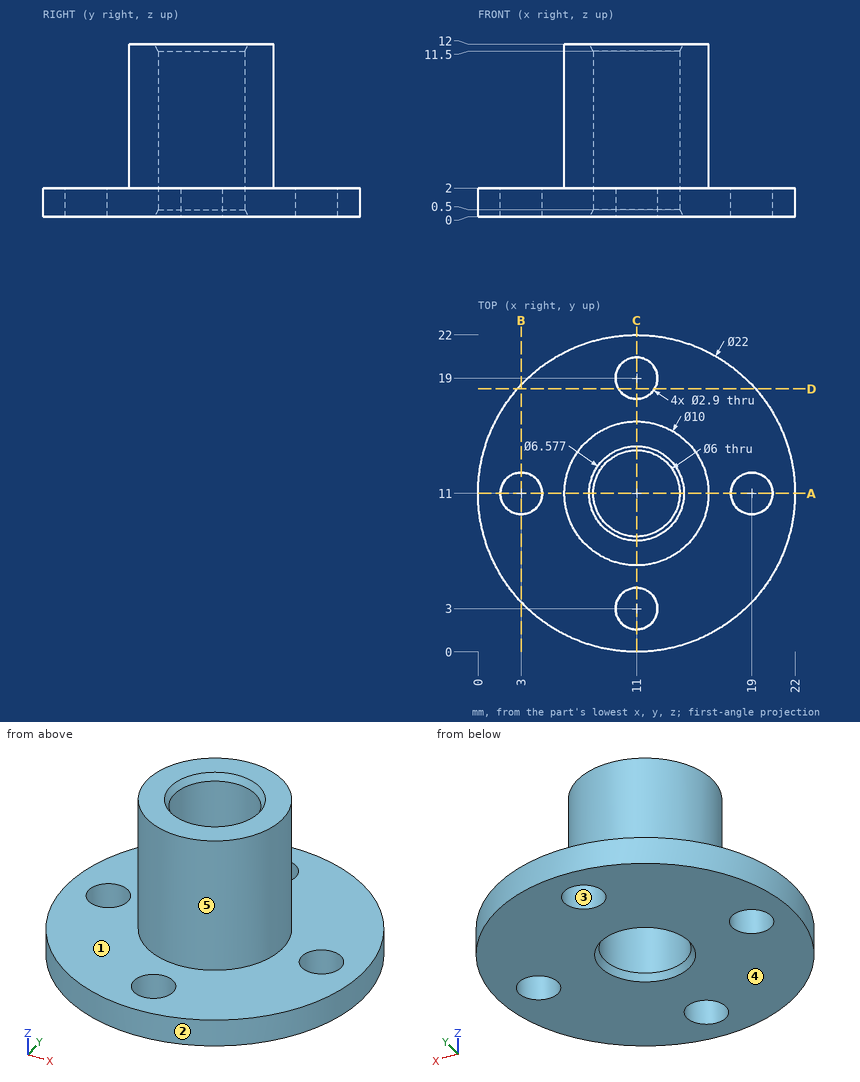
Can you work these out from the drawing? Everything is in mm from the part's minimum corner. A direction names the side the tool comes from. Coordinates: 2 decimals unless noted, no trailing zeros. Write each loop counter-clockwise with the first axis right and the second up, starting at its lowest first coordinate (ties: lowest second). Pieces come first, ordered by that corner, then holes. Notation, with made-up numbers: (23, 75.5) -> (54, 75.5) arc R25 ccw to (54, 94.5) -> close; hole circle Ø7 at (41.25, -13). An arc over 180 degrees is marked (long way). Write each question's results on one line, items separated by ' | '. Start each with the question number.
Item 1: If we section it at D-D, the plane y = 18.25: Write out the boundary of the cut face in (x, z).
Item 2: On a 3-axis mill with a long thin cutter (end or side, diameter ignored), from which of +Z, -Z, +X, -X, +Y, -Y can I reach the whole of each face in a straight line? I mean the marked faces 1 and 2. Say none if no direction works.
Item 3: I'm going to push flat-ended pins straight in: P1, Ø3, axis at x = 16, y = 11, coming from the -Z side; P2, Ø5, axis at y = 9.5, z = 10.5, coming from the +X side; P3, Ø3.5, axis at x = 11, y = 19, coming from the +Z side. Where does each tip first touch, or does it pass through?
Item 4: If we section it at B-B, the plane x = 3: Write out the boundary of the cut face in (y, z), and give its area (3 significant figures).
Item 5: Please list where these lines run through material, in increasing order: probe 1 along X at (y, z) = (11, 0.6); probe 2 along Y at (x, z) = (11, 6.5).
Item 6: Thinking about a two-plate mould opening in Y: for the marked faces 3, 4 and 5, which applies, released by +Y, released by -Y, zero draft, split by the parting line, or undercut?
Item 7: If we section it at A-A, the plane y = 11: Write out the boundary of the cut face in (x, z).
Answer block:
1) outline: (2.73, 0) -> (9.76, 0) -> (9.76, 2) -> (2.73, 2) -> close; (12.24, 0) -> (19.27, 0) -> (19.27, 2) -> (12.24, 2) -> close
2) face 1: +Z | face 2: +Z, -Z
3) P1: z = 0 | P2: x = 16 | P3: z = 2
4) outline: (3.45, 0) -> (9.55, 0) -> (9.55, 2) -> (3.45, 2) -> close; (12.45, 0) -> (18.55, 0) -> (18.55, 2) -> (12.45, 2) -> close | area: 24.4 mm²
5) probe 1: 0 to 1.55, 4.45 to 8, 14 to 17.55, 20.45 to 22 | probe 2: 6 to 8, 14 to 16
6) face 3: undercut | face 4: zero draft | face 5: split by the parting line
7) outline: (0, 0) -> (1.55, 0) -> (1.55, 2) -> (0, 2) -> close; (4.45, 0) -> (7.71, 0) -> (8, 0.5) -> (8, 11.5) -> (7.71, 12) -> (6, 12) -> (6, 2) -> (4.45, 2) -> close; (14, 0.5) -> (14.29, 0) -> (17.55, 0) -> (17.55, 2) -> (16, 2) -> (16, 12) -> (14.29, 12) -> (14, 11.5) -> close; (20.45, 0) -> (22, 0) -> (22, 2) -> (20.45, 2) -> close
